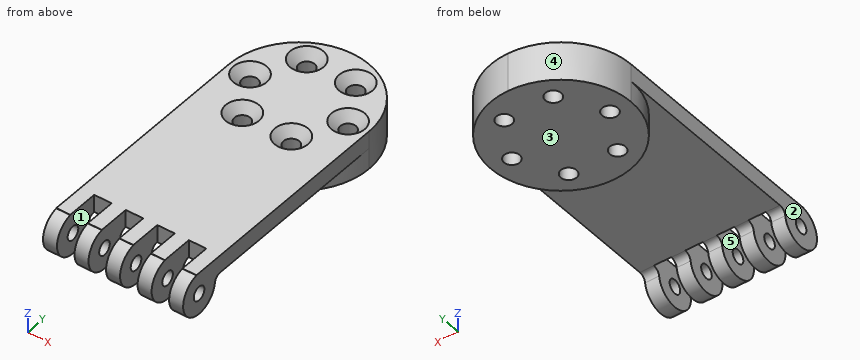
```python
from build123d import *

# Parameters (mm, degrees)
SKETCH7_W           = 40
SKETCH7_H           = 40
BOSS_EXTRUDE1_DEPTH = 11
SKETCH8_W           = 40
SKETCH8_H           = 5
BOSS_EXTRUDE2_DEPTH = 36
SKETCH10_R          = 2.25
CUT_EXTRUDE1_DEPTH  = 25
FILLET1_R           = 20
SKETCH11_W          = 4
SKETCH11_H          = 5
BOSS_EXTRUDE3_DEPTH = 9
SKETCH14_R          = 6
BOSS_EXTRUDE4_DEPTH = 4
LPATTERN1_COUNT     = 5
LPATTERN1_PITCH     = 9
SKETCH15_R          = 2
CUT_EXTRUDE2_DEPTH  = 82.369527466
CHAMFER1_SIZE       = 2.5
FILLET2_R           = 2


with BuildPart() as part:
    # Sketch7 → Boss-Extrude1 (new body)
    with BuildSketch(Plane.XY):
        Rectangle(SKETCH7_W, SKETCH7_H)
    extrude(amount=BOSS_EXTRUDE1_DEPTH)

    # Sketch8 → Boss-Extrude2 (add)
    with BuildSketch(Plane.XZ.offset(20)):
        with Locations((0, 8.5)):
            Rectangle(SKETCH8_W, SKETCH8_H)
    extrude(amount=BOSS_EXTRUDE2_DEPTH)

    # Sketch10 → Cut-Extrude1 (cut)
    with BuildSketch(Plane.XY.offset(11)):
        with Locations((-7.00009521, 12.124420806)):
            Circle(SKETCH10_R)
        with Locations((6.99990479, 12.124420806)):
            Circle(SKETCH10_R)
        with Locations((13.99990479, 6.5153e-05)):
            Circle(SKETCH10_R)
        with Locations((6.99990479, -12.1242905)):
            Circle(SKETCH10_R)
        with Locations((-7.00009521, -12.1242905)):
            Circle(SKETCH10_R)
        with Locations((-14.00009521, 6.5153e-05)):
            Circle(SKETCH10_R)
    extrude(amount=-CUT_EXTRUDE1_DEPTH, mode=Mode.SUBTRACT)

    # Fillet1
    fillet1_edges = [part.edges().sort_by_distance(p)[0] for p in [
        (20, -20, 3),
        (20, 20, 5.5),
        (-20, 20, 5.5),
        (-20, -20, 3),
    ]]
    fillet(fillet1_edges, radius=FILLET1_R - 0.0001)  # a hair under: the kernel refuses the full size

    # Sketch11 → Boss-Extrude3 (add)
    with BuildSketch(Plane.XZ.offset(56)):
        with Locations((-18, 8.5)):
            Rectangle(SKETCH11_W, SKETCH11_H)
    boss_extrude3 = extrude(amount=BOSS_EXTRUDE3_DEPTH)

    # Sketch14 → Boss-Extrude4 (add)
    with BuildSketch(Plane(origin=(-16, 0, 0), x_dir=(0, 0, -1), z_dir=(1, 0, 0))):
        with Locations((-5, -64)):
            Circle(SKETCH14_R)
    boss_extrude4 = extrude(amount=-BOSS_EXTRUDE4_DEPTH)

    # LPattern1: Boss-Extrude3, Boss-Extrude4 ×5
    with Locations(*[(i * LPATTERN1_PITCH, 0, 0) for i in range(1, LPATTERN1_COUNT)]):
        add(boss_extrude3)
        add(boss_extrude4)

    # Sketch15 → Cut-Extrude2 (cut, through all)
    with BuildSketch(Plane.ZY.offset(20)):
        with Locations(Location((5, -64, 0), (0, 0, 270))):
            Circle(SKETCH15_R)
    extrude(amount=-CUT_EXTRUDE2_DEPTH, mode=Mode.SUBTRACT)

    # Chamfer1
    chamfer1_edges = [part.edges().sort_by_distance(p)[0] for p in [
        (-16.25009521, 6.5153e-05, 11),
        (-9.25009521, -12.1242905, 11),
        (4.74990479, -12.1242905, 11),
        (11.74990479, 6.5153e-05, 11),
        (4.74990479, 12.124420806, 11),
        (-9.25009521, 12.124420806, 11),
    ]]
    chamfer(chamfer1_edges, length=CHAMFER1_SIZE)

    # Fillet2
    fillet2_edges = [part.edges().sort_by_distance(p)[0] for p in [
        (-18, -58.083920217, 6),
        (-9, -58.083920217, 6),
        (0, -58.083920217, 6),
        (9, -58.083920217, 6),
        (18, -58.083920217, 6),
    ]]
    fillet(fillet2_edges, radius=FILLET2_R)


solid = part.part
```
Verification items for the finished model (mm, model axes). Face numbers are marked on the shaded views. A direction names the side the tool comes from. Round coordinates to 2 decimals unless told otherwise and drop trailing zeros. Answer as a JSON object with one key per item and string values. Group by question number.
Q1. Thickness scan on line 1 (Y direction, x = 9, z = 6.25); line 2 (Y direction, x = 6.5, z = 9.25); line 3 (X direction, y = 1, z = 2). Record the ranges inside material, lowest first.
Q2. Section check A-A, the plane z = 1.25. Give the number of separate pieces and of enclosed holes in the cut face, plus the area to 3 significant figures.
Q3. Tool access check on the marked faces 1 and 2. Record the directions out of +Z, -Z, +X, -X, +Y, -Y that give a thin tool (end or side, any length) a straight path to the whole face; none if there is none.
Q4. Go/stop test with flat-tipped pins: pin 1 Ø5.5 at (x, z) = (12.5, 8.5) entering from -Y; pin 2 Ø6 at (x, y) = (-14, 0) entering from -Z; pin 3 Ø3 at (x, z) = (-2.5, 1) entering from -Y. Record where each tip stops, or that it passes through.
Q5. Mould release check, pull along X, two halves, no side actions. Record for the marked faces 3, 4 and 5: released by +X, released by -X, zero draft, split by the parting line, or undercut.
Found:
{
 "1": {"line 1": "y = -69.87 to -65.56, -62.44 to -13.15, -11.09 to 11.09, 13.16 to 17.86", "line 2": "y = -56 to -15.08, -9.17 to 9.17, 15.08 to 18.91", "line 3": "x = -19.97 to -16.02, -11.98 to 11.98, 16.02 to 19.97"},
 "2": {"separate pieces": "6", "enclosed holes": "6", "area": "1,350 mm^2"},
 "3": {"face 1": "+Z, -Z, -Y", "face 2": "+Z, -Z, -X, +Y, -Y"},
 "4": {"pin 1": "stops at y = -69.88", "pin 2": "stops at z = 0", "pin 3": "stops at y = -69.41"},
 "5": {"face 3": "zero draft", "face 4": "released by -X", "face 5": "undercut"}
}
